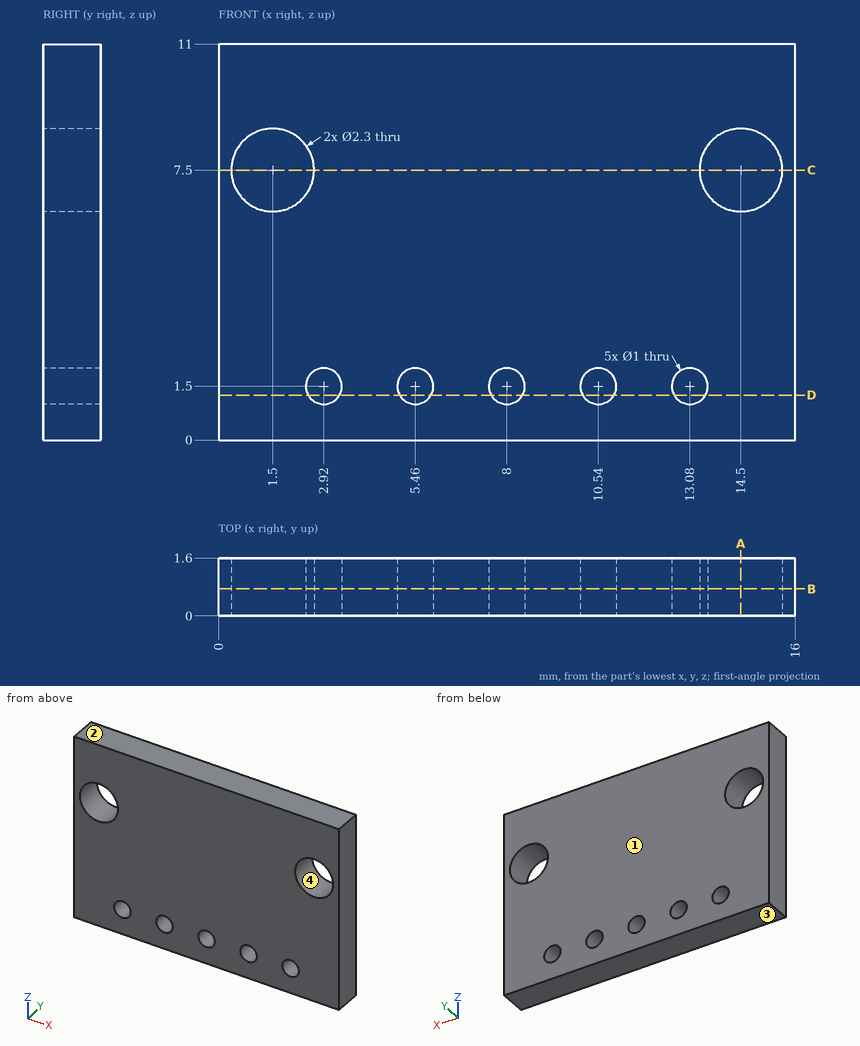
Geometry check sheet. Reference: drawing and pictorial views, mm from the part's lowest x, y, z. Give positions to 0.01 mm unless a question says otherwise; leave off trailing zeros. Loops run counter-clockwise (first coordinate to the right, second up) from the corner with the lowest first, then second, coordinate; pieces in that order, holes last. Notation, with made-up numbers: (-1, 38.25) - (9, 38.25) arc R35 ccw to (9, 70.25) - close; hole circle Ø1 at (89.25, -16.75). An arc over 180 degrees is marked (long way). Use CSV: the item, a comma, the result in double quotes. Start each with the question number.
Q1. Section check A-A, the plane x = 14.5. Record the cut outline in (y, z), and give its area (3 significant figures).
Q2. Scan lines: probe 1 along X at (y, z) = (1.15, 7.5); probe 2 along X at (y, z) = (1.15, 1.5); probe 3 along Z at (x, y) = (1.5, 0.8). Record each from-to range of solid material in increasing order. Write a range as from..to.
Q3. Section check B-B, the plane y = 0.75. Record the cut outline in (x, z).
Q4. Go/stop test with a flat-tipped pin: pin 1 Ø1.4 at (x, z) = (14.5, 7.5) entering from -Y. Record where the tip stops, or that it passes through.
Q5. Section check D-D, the plane z = 1.25. Record the cut outline in (x, y).
Q6. Release check for a two-part mould opening along Z. For the marked faces 1, 2, 3 and 4 record: +Z half, -Z half, draft (parallel to the pull), parting line (faces both ways), or undercut.
Q7. Section check C-C, the plane z = 7.5. Record the cut outline in (x, y).
Findings below:
1,outline,"(0, 0) - (1.6, 0) - (1.6, 6.35) - (0, 6.35) - close; (0, 8.65) - (1.6, 8.65) - (1.6, 11) - (0, 11) - close"
1,area,"13.9 mm^2"
2,probe 1,"x = 0..0.35, 2.65..13.35, 15.65..16"
2,probe 2,"x = 0..2.42, 3.42..4.96, 5.96..7.5, 8.5..10.04, 11.04..12.58, 13.58..16"
2,probe 3,"z = 0..6.35, 8.65..11"
3,outline,"(0, 0) - (16, 0) - (16, 11) - (0, 11) - close; hole circle Ø2.3 at (1.5, 7.5); hole circle Ø1 at (2.92, 1.5); hole circle Ø1 at (5.46, 1.5); hole circle Ø1 at (8, 1.5); hole circle Ø1 at (10.54, 1.5); hole circle Ø1 at (13.08, 1.5); hole circle Ø2.3 at (14.5, 7.5)"
4,pin 1,"passes through"
5,outline,"(0, 0) - (2.49, 0) - (2.49, 1.6) - (0, 1.6) - close; (3.35, 0) - (5.03, 0) - (5.03, 1.6) - (3.35, 1.6) - close; (5.89, 0) - (7.57, 0) - (7.57, 1.6) - (5.89, 1.6) - close; (8.43, 0) - (10.11, 0) - (10.11, 1.6) - (8.43, 1.6) - close; (10.97, 0) - (12.65, 0) - (12.65, 1.6) - (10.97, 1.6) - close; (13.51, 0) - (16, 0) - (16, 1.6) - (13.51, 1.6) - close"
6,face 1,"draft"
6,face 2,"+Z half"
6,face 3,"-Z half"
6,face 4,"undercut"
7,outline,"(0, 0) - (0.35, 0) - (0.35, 1.6) - (0, 1.6) - close; (2.65, 0) - (13.35, 0) - (13.35, 1.6) - (2.65, 1.6) - close; (15.65, 0) - (16, 0) - (16, 1.6) - (15.65, 1.6) - close"
